For this review, use the dimensioned drawing (mm, ordinates from the lowest corner) and the shaded views. A direction names the side the tool comes from. Round coordinates to 2 decimals unless told otherwise and drop trailing zeros. Loops run counter-clockwise (first coordinate to the right, second up) from the corner with the lowest first, then second, coordinate; pieces in that order, holes last. Notation, with made-up numbers: (4.5, -35) -> (19.5, -35) arc R9 ccw to (19.5, -23) -> close; hole circle Ø6 at (55.25, 0.25). An arc over 180 degrees is marked (long way). Write each question's results on one line, items separated by ' | '. Start each with the question number.
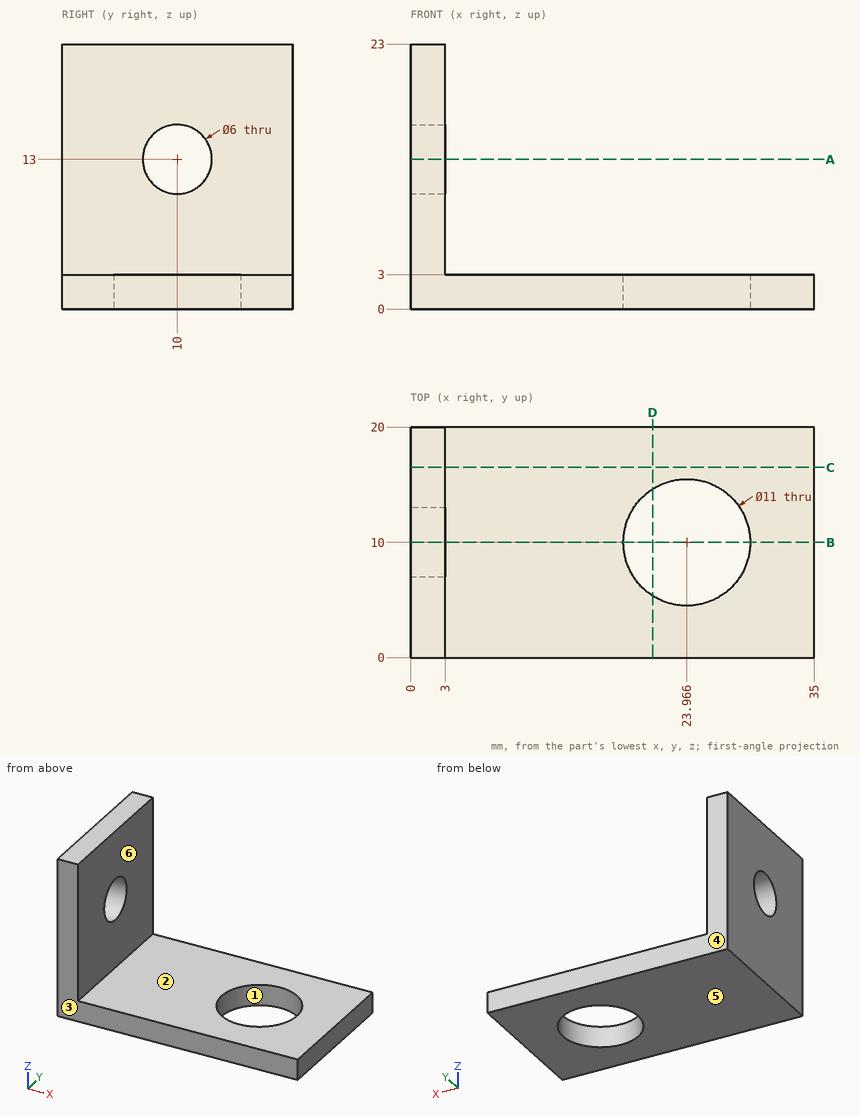
1) Take a section at C-C (y = 16.5). Write out the cut boundary in (x, z), plus the area to 3 significant figures.
2) Take a section at D-D (x = 21). Write out the cut boundary in (y, z).
3) For the marked faces 5 and 6, list the 3-axis set-ups (+Z, -Z, +X, -X, +Y, -Y) from which the entire face can be reached by the end or side of a thin tool; tool diameter is ignored.
4) Take a section at B-B (y = 10). Write out the cut boundary in (x, z).
5) The part is to be moulded in two halves that separate along Y. For the marked faces 1, 2, 3 and 4, say which applies: +Y half, -Y half, draft (parallel to the pull), parting line (faces both ways), or undercut.
6) Take a section at A-A (z = 13). Write out the cut boundary in (x, y).
7) To check wall thickness, follow line 1 (Z direction, x = 0.95, y = 10); line 2 (Z direction, x = 31, y = 8.5). State the ranges of each line that lie inside material, in increasing order. Write a range as from..to.
8) Insertion check: pin 1 (1.5 mm diameter, centred on x = 4, y = 11.5, fed in from -Z); pin 2 (10 mm diameter, centred on y = 6, z = 14.5, fed in from +X); pin 3 (4 mm diameter, centred on x = 27, y = 12.5, fed in from +Z). Each pin has a flat end and moves straight along its axis. Give the tip position at first contact, or say it passes through.
Geometry check:
1) outline: (0, 0) -> (35, 0) -> (35, 3) -> (3, 3) -> (3, 23) -> (0, 23) -> close | area: 165 mm^2
2) outline: (0, 0) -> (5.37, 0) -> (5.37, 3) -> (0, 3) -> close; (14.63, 0) -> (20, 0) -> (20, 3) -> (14.63, 3) -> close
3) face 5: -Z, +X, -X, +Y, -Y | face 6: +Z, +X, +Y, -Y
4) outline: (0, 0) -> (18.47, 0) -> (18.47, 3) -> (3, 3) -> (3, 10) -> (0, 10) -> close; (0, 16) -> (3, 16) -> (3, 23) -> (0, 23) -> close; (29.47, 0) -> (35, 0) -> (35, 3) -> (29.47, 3) -> close
5) face 1: undercut | face 2: draft | face 3: -Y half | face 4: +Y half
6) outline: (0, 0) -> (3, 0) -> (3, 7) -> (0, 7) -> close; (0, 13) -> (3, 13) -> (3, 20) -> (0, 20) -> close
7) line 1: z = 0..10, 16..23 | line 2: z = 0..3
8) pin 1: stops at z = 0 | pin 2: stops at x = 3 | pin 3: stops at z = 3
